from build123d import *

# Parameters (mm, degrees)
BOSS_EXTRUDE1_DEPTH = 3.5814
SKETCH2_R           = 1.45
CUT_EXTRUDE1_DEPTH  = 4.5814
BOSS_EXTRUDE2_DEPTH = 3.5814


with BuildPart() as part:
    # Sketch1 → Boss-Extrude1 (new body)
    with BuildSketch(Plane(origin=(0, 0, 0), x_dir=(1, 0, 0), z_dir=(0, 1, 0))):
        Polygon((-22.5, -17.05), (22.5, -17.05), (22.5, -2.05), (1.7907, -2.05), (1.7907, 2.05), (9.398, 2.05), (1.7907, 7.13), (-1.7907, 7.13), (-9.398, 2.05), (-1.7907, 2.05), (-1.7907, -2.05), (-22.5, -2.05), align=None)
    extrude(amount=BOSS_EXTRUDE1_DEPTH)

    # Sketch2 → Cut-Extrude1 (cut, through all)
    with BuildSketch(Plane(origin=(0, 3.5814, 0), x_dir=(1, 0, 0), z_dir=(0, 1, 0))):
        with Locations((-18.49, -9.55)):
            Circle(SKETCH2_R)
        with Locations((18.49, -9.55)):
            Circle(SKETCH2_R)
    extrude(amount=-CUT_EXTRUDE1_DEPTH, mode=Mode.SUBTRACT)

    # Sketch3 → Boss-Extrude2 (add)
    with BuildSketch(Plane(origin=(0, 3.5814, 0), x_dir=(1, 0, 0), z_dir=(0, 1, 0))):
        Polygon((1.7907, 18.56), (9.398, 13.48), (9.398, 2.05), (1.7907, 7.13), (-1.7907, 7.13), (-9.398, 2.05), (-9.398, 13.48), (-1.7907, 18.56), align=None)
    extrude(amount=-BOSS_EXTRUDE2_DEPTH)


solid = part.part
The model under review builds one solid part; all positions refer to its coordinate system, in mm. A direction names the side the tool comes from. Round coordinates to 2 decimals unless told otherwise and drop trailing zeros. Write each loop counter-clockwise with the first axis right and the second up, starting at its lowest first coordinate (ties: lowest second). Pieces come first, ordered by that corner, then holes. Notation, with made-up numbers: (18.5, 80.25) - (23.5, 80.25) arc R17 ccw to (23.5, 91.25) - close; hole circle Ø6 at (-19.5, 47.5). An arc over 180 degrees is marked (long way). One line per item, written item: value. Start each with the question number.
1. Clearance check with flat-ended pins moving along their axes: P1, Ø2, axis at y = 0.5, z = -11, coming from the -X side; P2, Ø1.8, axis at y = 1.5, z = -8.5, coming from the +X side; P3, Ø1.8, axis at y = 2, z = -0.5, coming from the -X side. State where each tip first meets the part, or that it passes through.
2. The part is to be moulded in two halves that separate along Z. For faces 1 (the face through (0, 0, 3)), 2 (the face through (12, 2, 2.05)), 3 (the face through (-5.648, 1.816, -15.984)), say which applies: released by +Z, released by -Z, zero draft, split by the parting line, or undercut.
3. Machinability: for faces 4 (the face through (-6, 2, -2.05)), 5 (the face through (9.398, 2, -8)), 6 (the face through (6, 2, -2.05)), 7 (the face through (-9.398, 2, -8)), which of the approach directions +Z, -Z, +X, -X, +Y, -Y give a long, thin tool a straight path to every point of the face, cutting with its end or side? Answer none if there is none.
4. To check wall thickness, follow L1, parallel to X at y = 1.9, z = 9.55; L2, parallel to Z at x = -18.49, y = 1.3; L3, parallel to X at y = 1.05, z = 9. State the ranges of each line that lie inside material, in increasing order. Write a range as from..to.
5. Consider section C-C on y = 2.1. Write out the cut boundary in (x, z).
6. Consider section A-A on z = 9.55. Write out the cut boundary in (x, y), and give its area (3 significant figures).
7. Consider section B-B on x = 18.49. Write out the cut boundary in (y, z), and give its area (3 significant figures).
8. Consider section D-D on x = -7. Write out the cut boundary in (y, z), and give its area (3 significant figures).
Checks:
1. P1: stops at x = -9.4
1. P2: stops at x = 9.4
1. P3: stops at x = -1.79
2. face 1: zero draft
2. face 2: undercut
2. face 3: released by -Z
3. face 4: -X, +Y, -Y
3. face 5: -Z, +X, +Y, -Y
3. face 6: +X, +Y, -Y
3. face 7: -Z, -X, +Y, -Y
4. L1: x = -22.5..-19.94, -17.04..17.04, 19.94..22.5
4. L2: z = 2.05..8.1, 11..17.05
4. L3: x = -22.5..-19.83, -17.15..17.15, 19.83..22.5
5. outline: (-22.5, 2.05) - (-1.79, 2.05) - (-1.79, -2.05) - (-9.4, -2.05) - (-9.4, -13.48) - (-1.79, -18.56) - (1.79, -18.56) - (9.4, -13.48) - (9.4, -2.05) - (1.79, -2.05) - (1.79, 2.05) - (22.5, 2.05) - (22.5, 17.05) - (-22.5, 17.05) - close; hole circle Ø2.9 at (-18.49, 9.55); hole circle Ø2.9 at (18.49, 9.55)
6. outline: (-22.5, 0) - (-19.94, 0) - (-19.94, 3.58) - (-22.5, 3.58) - close; (-17.04, 0) - (17.04, 0) - (17.04, 3.58) - (-17.04, 3.58) - close; (19.94, 0) - (22.5, 0) - (22.5, 3.58) - (19.94, 3.58) - close
6. area: 140 mm^2
7. outline: (0, 2.05) - (3.58, 2.05) - (3.58, 8.1) - (0, 8.1) - close; (0, 11) - (3.58, 11) - (3.58, 17.05) - (0, 17.05) - close
7. area: 43.3 mm^2
8. outline: (0, -15.08) - (3.58, -15.08) - (3.58, -2.05) - (0, -2.05) - close; (0, 2.05) - (3.58, 2.05) - (3.58, 17.05) - (0, 17.05) - close
8. area: 100 mm^2
